Can you work these out from the model? Positions are in its coordinate system, mm. Face numbers are marked on the shaded views. A direction names the side the tool comes from. Round coordinates to 2 decimals unless told otherwise and drop trailing zeros. Loops run counter-clockwise (first coordinate to the right, second up) from the corner with the lowest first, then second, coordinate; pieces in that order, holes last. Notation, with made-up numbers: M 73,54 L 87,54 A23 cw 87,80 Z; hole C -21,76.5 d5. An arc over 180 degrees is marked long. Return JSON: item names as keys, results as strings.
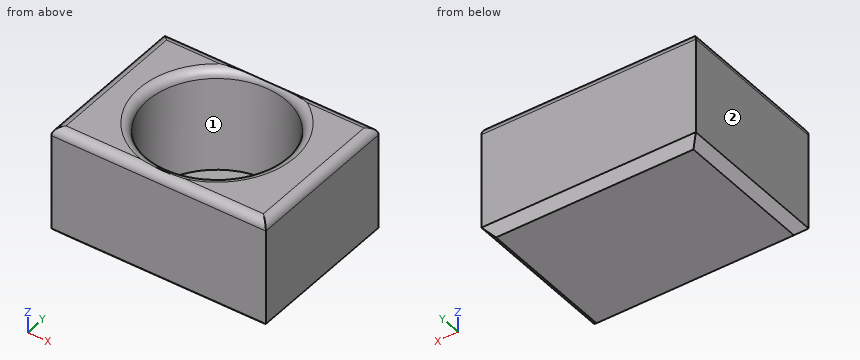
```python
from build123d import *

# Parameters (mm, degrees)
F0_W        = 125.5629397929
F0_H        = 91.4415977895
F0_R        = 40.6040371895
F1_DEPTH    = 60
F2_W        = 118.2770989835
F2_H        = 87.5040702522
F3_DEPTH    = 6
F4_T1_DEPTH = 150.5629397929
F4_T3_DEPTH = 116.4415977895
F5_SIZE     = 5


# Not quite as in the source:
# - a fillet or chamfer that OpenCascade refuses, or shapes differently, is made with other operations: its cross-section is extruded or revolved along the edge and cut away or added


with BuildPart() as f1:
    # F0 (on Top) → F1 (new body)
    with BuildSketch(Plane.XY):
        with Locations((1.0034125298, -8.6029302329)):
            Rectangle(F0_W, F0_H)
        with Locations((0, -5.6129307486)):
            Circle(F0_R, mode=Mode.SUBTRACT)
    extrude(amount=F1_DEPTH)

    # F2 (on face) → F3 (join)
    with BuildSketch(Plane(origin=(0, 0, 0), x_dir=(1, 0, 0), z_dir=(0, 0, -1))):
        Polygon((63.7848824263, -37.1178686619), (63.7848824263, 54.3237291276), (-61.7780573666, 54.3237291276), (-61.7780573666, -37.1178686619), (-58.5906021297, -37.1178686619), (-58.5906021297, 50.3862015903), (59.6864968538, 50.3862015903), (59.6864968538, -37.1178686619), align=None)
        with Locations((0.5479473621, 6.6341664642)):
            Rectangle(F2_W, F2_H)
    extrude(amount=F3_DEPTH)

    # F4: fillet of radius 5 on 5 edges, made by hand

    # F4_s2 → F4_t1 (cut)
    with BuildSketch(Plane.YZ.offset(-74.2780573666)):
        with BuildLine():
            ThreePointArc((37.1178686619, 55), (35.6534025678, 58.5355339059), (32.1178686619, 60))
            Line((32.1178686619, 60), (37.1178686619, 60))
            Line((37.1178686619, 60), (37.1178686619, 55))
        make_face()
        with BuildLine():
            ThreePointArc((-49.3237291276, 60), (-52.8592630336, 58.5355339059), (-54.3237291276, 55))
            Line((-54.3237291276, 55), (-54.3237291276, 60))
            Line((-54.3237291276, 60), (-49.3237291276, 60))
        make_face()
    extrude(amount=F4_T1_DEPTH, mode=Mode.SUBTRACT)

    # F4_s4 → F4_t3 (cut)
    with BuildSketch(Plane.XZ.offset(-49.6178686619)):
        with BuildLine():
            ThreePointArc((63.7848824263, 55), (62.3204163322, 58.5355339059), (58.7848824263, 60))
            Line((58.7848824263, 60), (63.7848824263, 60))
            Line((63.7848824263, 60), (63.7848824263, 55))
        make_face()
        with BuildLine():
            ThreePointArc((-61.7780573666, 55), (-60.3135912725, 58.5355339059), (-56.7780573666, 60))
            Line((-56.7780573666, 60), (-61.7780573666, 60))
            Line((-61.7780573666, 60), (-61.7780573666, 55))
        make_face()
    extrude(amount=F4_T3_DEPTH, mode=Mode.SUBTRACT)

    # F4_s5 → F4_t6 (revolve, cut)
    with BuildSketch(Plane.XZ.offset(5.6129307486)):
        with BuildLine():
            ThreePointArc((45.6040371895, 60), (42.0685032836, 58.5355339059), (40.6040371895, 55))
            Line((40.6040371895, 55), (40.6040371895, 60))
            Line((40.6040371895, 60), (45.6040371895, 60))
        make_face()
    revolve(axis=Axis((0, -5.6129307486, 60), (0, 0, 1)), mode=Mode.SUBTRACT)

    # F5
    f5_edges = [f1.edges().sort_by_distance(p)[0] for p in [
        (1.003413, 37.117869, -6),
        (63.784882, -8.60293, -6),
        (1.003413, -54.323729, -6),
        (-61.778057, -8.60293, -6),
    ]]
    chamfer(f5_edges, length=F5_SIZE)


solid = f1.part
```
Q1. I'm going to push a flat-ended pin straight in: pin 1 Ø5 at (x, y) = (16.5, -9) entering from +Z. Where does the tip first touch, or does it pass through?
Results:
{"pin 1": "stops at z = 0"}
Q2. On a 3-axis mill with a long thin cutter (end or side, diameter ignored), from which of +Z, -Z, +X, -X, +Y, -Y can I reach the whole of each face in a straight line? I mean the marked faces 1 and 2. Say none if no direction works.
Results:
{"face 1": "+Z", "face 2": "+Z, -Z, -X, +Y, -Y"}
Q3. Suppose I cut it at A-A, the plane z = 12. Please give me the cut outline in (x, y).
Results:
{"outline": "M -61.78,-54.32 L 63.78,-54.32 L 63.78,37.12 L -61.78,37.12 Z; hole C 0,-5.61 d81.21"}
Q4. If I drill on line 1 along Y through (x, z) = (0, 37); line 2 along X through (y, z) = (-7, 12); line 3 along X through (y, z) = (-30.5, 18), over which ranges is the centre line in solid material (lowest first)?
Results:
{"line 1": "y = -54.32 to -46.22, 34.99 to 37.12", "line 2": "x = -61.78 to -40.58, 40.58 to 63.78", "line 3": "x = -61.78 to -32.08, 32.08 to 63.78"}
Q5. Suppose I cut it at B-B, the plane x = 0. Please give me the cut outline in (y, z), plus the area to 3 significant figures.
Results:
{"outline": "M -54.32,-1 L -49.32,-6 L 32.12,-6 L 37.12,-1 L 37.12,55 A5 ccw 36.05,58.08 A5 ccw 34.99,55 L 34.99,0 L -46.22,0 L -46.22,55 A5 ccw -50.27,59.91 A5 ccw -54.32,55 Z", "area": "1,120 mm2"}
